```python
from build123d import *

# Parameters (mm, degrees)
EXTRUDE_1_DEPTH     = 1000
EXTRUDE_START       = -400
EXTRUDE_3_DEPTH     = 370
EXTRUDE_START_2     = -50
EXTRUDE_4_DEPTH     = 20
CUT_EXTRUDE_START   = -20
CUT_EXTRUDE_1_DEPTH = 20
SKETCH_8_R          = 2.7
CUT_EXTRUDE_4_DEPTH = 2
SKETCH_9_R          = 1.25
CUT_EXTRUDE_5_DEPTH = 6
SKETCH_10_R         = 2.7
CUT_EXTRUDE_6_DEPTH = 2
SKETCH_11_R         = 1.25
CUT_EXTRUDE_7_DEPTH = 6


with BuildPart() as part:
    # 草图1 → 凸台-拉伸1 (new body)
    with BuildSketch(Plane(origin=(0, 0, 0), x_dir=(1, 0, 0), z_dir=(0, 1, 0))):
        with BuildLine():
            Line((-45, 0), (-42.5, 0))
            ThreePointArc((-42.5, 0), (0, 42.5), (42.5, 0))
            Line((42.5, 0), (45, 0))
            ThreePointArc((45, 0), (0, 45), (-45, 0))
        make_face()
    extrude(amount=EXTRUDE_1_DEPTH)

    # 草图3 → 凸台-拉伸3 (add)
    with BuildSketch(Plane(origin=(0, 1000, 0), x_dir=(1, 0, 0), z_dir=(0, 1, 0)).offset(EXTRUDE_START)):
        with BuildLine():
            Line((-31.337456942, 24.046076446), (-33.717516962, 25.872360733))
            ThreePointArc((-33.717516962, 25.872360733), (-30.0520382, 30.0520382), (-25.872360733, 33.717516962))
            Line((-25.872360733, 33.717516962), (-24.046076446, 31.337456942))
            ThreePointArc((-24.046076446, 31.337456942), (-27.930717857, 27.930717857), (-31.337456942, 24.046076446))
        make_face()
        with BuildLine():
            Line((24.046076446, 31.337456942), (25.872360733, 33.717516962))
            ThreePointArc((25.872360733, 33.717516962), (30.0520382, 30.0520382), (33.717516962, 25.872360733))
            Line((33.717516962, 25.872360733), (31.337456942, 24.046076446))
            ThreePointArc((31.337456942, 24.046076446), (27.930717857, 27.930717857), (24.046076446, 31.337456942))
        make_face()
    extrude(amount=EXTRUDE_3_DEPTH)

    # 草图4 → 凸台-拉伸4 (add)
    with BuildSketch(Plane(origin=(0, 1000, 0), x_dir=(1, 0, 0), z_dir=(0, 1, 0)).offset(EXTRUDE_START_2)):
        with BuildLine():
            Line((-37.671819555, 11.87787908), (-40.532970407, 12.779996479))
            ThreePointArc((-40.532970407, 12.779996479), (-39.962245398, 14.466130884), (-39.321413031, 16.12688678))
            Line((-39.321413031, 16.12688678), (-36.545783876, 14.988518301))
            ThreePointArc((-36.545783876, 14.988518301), (-37.141381017, 13.444992233), (-37.671819555, 11.87787908))
        make_face()
        with BuildLine():
            Line((36.545783876, 14.988518301), (39.321413031, 16.12688678))
            ThreePointArc((39.321413031, 16.12688678), (39.962245398, 14.466130884), (40.532970407, 12.779996479))
            Line((40.532970407, 12.779996479), (37.671819555, 11.87787908))
            ThreePointArc((37.671819555, 11.87787908), (37.141381017, 13.444992233), (36.545783876, 14.988518301))
        make_face()
        with BuildLine():
            Line((11.87787908, 37.671819555), (12.779996479, 40.532970407))
            ThreePointArc((12.779996479, 40.532970407), (14.466130884, 39.962245398), (16.12688678, 39.321413031))
            Line((16.12688678, 39.321413031), (14.988518301, 36.545783876))
            ThreePointArc((14.988518301, 36.545783876), (13.444992233, 37.141381017), (11.87787908, 37.671819555))
        make_face()
        with BuildLine():
            Line((-14.988518301, 36.545783876), (-16.12688678, 39.321413031))
            ThreePointArc((-16.12688678, 39.321413031), (-14.466130884, 39.962245398), (-12.779996479, 40.532970407))
            Line((-12.779996479, 40.532970407), (-11.87787908, 37.671819555))
            ThreePointArc((-11.87787908, 37.671819555), (-13.444992233, 37.141381017), (-14.988518301, 36.545783876))
        make_face()
    extrude(amount=EXTRUDE_4_DEPTH)

    # 草图5 → 切除-拉伸1 (cut)
    with BuildSketch(Plane(origin=(0, 970, 0), x_dir=(1, 0, 0), z_dir=(0, 1, 0)).offset(CUT_EXTRUDE_START)):
        with BuildLine():
            Line((-38.293502312, 13.185510256), (-40.184539463, 13.836646564))
            ThreePointArc((-40.184539463, 13.836646564), (-39.769465933, 14.987981166), (-39.321413031, 16.12688678))
            Line((-39.321413031, 16.12688678), (-37.444114361, 15.433350242))
            ThreePointArc((-37.444114361, 15.433350242), (-37.885483249, 14.315731173), (-38.293502312, 13.185510256))
        make_face()
        with BuildLine():
            Line((-15.433350242, 37.444114361), (-16.12688678, 39.321413031))
            ThreePointArc((-16.12688678, 39.321413031), (-14.987981166, 39.769465933), (-13.836646564, 40.184539463))
            Line((-13.836646564, 40.184539463), (-13.185510256, 38.293502312))
            ThreePointArc((-13.185510256, 38.293502312), (-14.315731173, 37.885483249), (-15.433350242, 37.444114361))
        make_face()
        with BuildLine():
            Line((13.185510256, 38.293502312), (13.836646564, 40.184539463))
            ThreePointArc((13.836646564, 40.184539463), (14.987981166, 39.769465933), (16.12688678, 39.321413031))
            Line((16.12688678, 39.321413031), (15.433350242, 37.444114361))
            ThreePointArc((15.433350242, 37.444114361), (14.315731173, 37.885483249), (13.185510256, 38.293502312))
        make_face()
        with BuildLine():
            Line((37.444114361, 15.433350242), (39.321413031, 16.12688678))
            ThreePointArc((39.321413031, 16.12688678), (39.769465933, 14.987981166), (40.184539463, 13.836646564))
            Line((40.184539463, 13.836646564), (38.293502312, 13.185510256))
            ThreePointArc((38.293502312, 13.185510256), (37.885483249, 14.315731173), (37.444114361, 15.433350242))
        make_face()
    extrude(amount=CUT_EXTRUDE_1_DEPTH, mode=Mode.SUBTRACT)

    # 草图8 → 切除-拉伸4 (cut)
    with BuildSketch(Plane(origin=(-31.819805153, 0, -31.819805153), x_dir=(0, -1, 0), z_dir=(-0.7071067811865488, 0, -0.7071067811865464))):
        with Locations(Location((-980, 0, 0), (0, 0, 90))):
            Circle(SKETCH_8_R)
    extrude(amount=-CUT_EXTRUDE_4_DEPTH, mode=Mode.SUBTRACT)

    # 草图9 → 切除-拉伸5 (cut)
    with BuildSketch(Plane(origin=(-31.819805153, 0, -31.819805153), x_dir=(0, -1, 0), z_dir=(-0.7071067811865488, 0, -0.7071067811865464))):
        with Locations(Location((-980, 0, 0), (0, 0, 90))):
            Circle(SKETCH_9_R)
    extrude(amount=-CUT_EXTRUDE_5_DEPTH, mode=Mode.SUBTRACT)

    # 草图10 → 切除-拉伸6 (cut)
    with BuildSketch(Plane(origin=(31.819805153, 0, -31.819805153), x_dir=(0, -1, 0), z_dir=(0.7071067811865488, 0, -0.7071067811865464))):
        with Locations(Location((-980, 0, 0), (0, 0, 90))):
            Circle(SKETCH_10_R)
    extrude(amount=-CUT_EXTRUDE_6_DEPTH, mode=Mode.SUBTRACT)

    # 草图11 → 切除-拉伸7 (cut)
    with BuildSketch(Plane(origin=(31.819805153, 0, -31.819805153), x_dir=(0, -1, 0), z_dir=(0.7071067811865488, 0, -0.7071067811865464))):
        with Locations(Location((-980, 0, 0), (0, 0, 90))):
            Circle(SKETCH_11_R)
    extrude(amount=-CUT_EXTRUDE_7_DEPTH, mode=Mode.SUBTRACT)


solid = part.part
```
Work out the finished part from the listing and answer in its coordinate system (mm). Round coordinates to 2 decimals unless told otherwise and drop trailing zeros. Write each loop counter-clockwise with the first axis right and the second up, starting at its lowest first coordinate (ties: lowest second). Pieces come first, ordered by that corner, then holes. Notation, with made-up numbers: (26.5, 29.5) -> (69.5, 29.5) arc R20 cw to (69.5, 49.5) -> close; hole circle Ø6 at (-13.5, -28). An arc over 180 degrees is marked (long way). Write each question's results on one line, items separated by ' | '.
1) The part is cut by section A-A (y = 890). Write down the section's boundary in (x, z).
Findings:
outline: (-45, 0) arc R45 ccw to (45, 0) -> (42.5, 0) arc R42.5 cw to (33.72, -25.87) -> (31.34, -24.05) arc R39.5 cw to (24.05, -31.34) -> (25.87, -33.72) arc R42.5 cw to (-25.87, -33.72) -> (-24.05, -31.34) arc R39.5 cw to (-31.34, -24.05) -> (-33.72, -25.87) arc R42.5 cw to (-42.5, 0) -> close
2) The part is cut by section B-B (x = 0). Write down the section's boundary in (y, z), and give its area (3 significant figures).
Findings:
outline: (0, -45) -> (1000, -45) -> (1000, -42.5) -> (0, -42.5) -> close | area: 2,500 mm²
3) The part is cut by section C-C (y = 69). Write down the section's boundary in (x, z).
Findings:
outline: (-45, 0) arc R45 ccw to (45, 0) -> (42.5, 0) arc R42.5 cw to (-42.5, 0) -> close
4) Flat-ended cylindrical pins translate along their axes: pin 1 (1 mm diameter, centred on x = 13, z = -38.5, fed in from -Y); pin 2 (1 mm diameter, centred on y = 387.5, z = -16, fed in from -X); pin 3 (12 mm diameter, centred on x = -8, y = 341.5, fed in from -Z). Find the tip coordinate at first contact, or state that the pin passes through.
Findings:
pin 1: stops at y = 950 | pin 2: stops at x = -42.25 | pin 3: stops at z = -44.96
5) Consider line 1 along X through (y, z) = (611, -34); line 2 along X through (y, z) = (135, -13); line 3 along Z through (x, y) = (17.5, 603). Determine where each line is inside the solid, lowest interval first. Write a range as [from, to].
Findings:
line 1: x = [-29.48, -25.5], [25.5, 29.48] | line 2: x = [-43.08, -40.46], [40.46, 43.08] | line 3: z = [-41.46, -38.73]
